Could you check a few things on this drawing? It's one solid part, dimensions in mm from its lowest x, y, z. A direction names the side the tool comes from. Coordinates: 2 decimals unless noted, no trailing zeros. Write each loop counter-clockwise with the first axis right and the second up, starting at its lowest first coordinate (ties: lowest second). Pieces come first, ordered by that corner, then holes. Notation, with made-up numbers: (-8.5, 37) - (9.5, 37) arc R18 ccw to (9.5, 68) - close; hole circle Ø3 at (77.5, -24). An arc over 180 degrees is marked (long way). Answer as a JSON object with one key per item and string values. Group by question number.
1) If we section it at B-B (x = 2): Write out the boundary of the cut face in (y, z).
2) Please list where these lines run through material, in increasing order: line 1 along Y through (x, z) = (4, 6.25); line 2 along Z through (x, y) = (4.5, 47); line 3 along Z through (x, y) = (4, 56).
3) On a 3-axis mill with a long thin cutter (end or side, diameter ignored), from which of +Z, -Z, +X, -X, +Y, -Y can I reach the whole of each face in a straight line? I mean the marked faces 1, 2 and 3. Say none if no direction works.
4) If we section it at A-A (z = 4.25): Write out the boundary of the cut face in (x, y).
5) If we section it at C-C (y = 16.5): Write out the boundary of the cut face in (x, z) (3 decimals), plus the area to 3 significant figures.
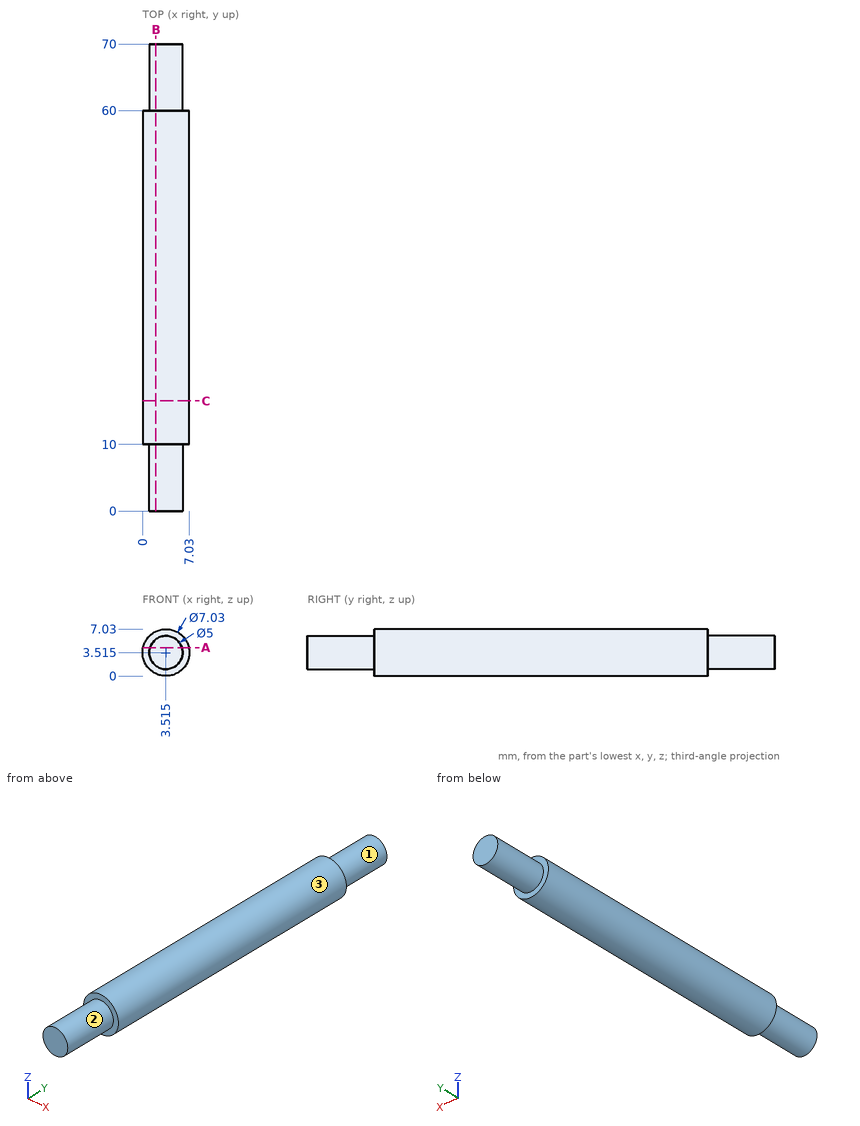
Here are the results:
{
 "1": {"outline": "(0, 1.53) - (10, 1.53) - (10, 0.34) - (60, 0.34) - (60, 1.53) - (70, 1.53) - (70, 5.5) - (60, 5.5) - (60, 6.69) - (10, 6.69) - (10, 5.5) - (0, 5.5) - close"},
 "2": {"line 1": "y = 10 to 60", "line 2": "z = 0.14 to 6.89", "line 3": "z = 0.03 to 7"},
 "3": {"face 1": "+Y", "face 2": "-Y", "face 3": "+Y, -Y"},
 "4": {"outline": "(0.08, 10) - (1.13, 10) - (1.13, 0) - (5.9, 0) - (5.9, 10) - (6.95, 10) - (6.95, 60) - (5.9, 60) - (5.9, 70) - (1.13, 70) - (1.13, 60) - (0.08, 60) - close"},
 "5": {"outline": "circle Ø7.03 at (3.515, 3.515)", "area": "38.8 mm²"}
}
